from build123d import *

# Parameters (mm, degrees)
PAD009_DEPTH    = 3
POCKET012_DEPTH = 5
SKETCH044_R     = 1.45
POCKET016_DEPTH = 22
FILLET007_R     = 1.5
FILLET015_R     = 0.5


with BuildPart() as part:
    # Sketch032 → Pad009 (new body)
    with BuildSketch(Plane.XY):
        with BuildLine():
            add(Edge.make_bspline(
                [(48.133333, -17.5342), (72.566704, -17.735607), (107.262527, -17.223288), (153.231854, -38.154949)],
                knots=[0, 0, 0, 0, 1, 1, 1, 1], degree=3))
            Line((153.231854, -38.154949), (175.310198, 11.234895))
            add(Edge.make_bspline(
                [(150.875, 88.9625), (150.875, 42.8625), (150.875, 22.157965), (175.310198, 11.234895)],
                knots=[0, 0, 0, 0, 1, 1, 1, 1], degree=3))
            add(Edge.make_bspline(
                [(85.725, 98.4875), (104.775, 98.4875), (104.775, 88.9625), (150.875, 88.9625)],
                knots=[0, 0, 0, 0, 1, 1, 1, 1], degree=3))
            Line((85.725, 98.4875), (66.675, 98.4875))
            add(Edge.make_bspline(
                [(66.675, 98.4875), (58.346897, 98.489647), (52.856461, 97.147667), (48.133333, 95.467873)],
                knots=[0, 0, 0, 0, 1, 1, 1, 1], degree=3))
            Line((48.133333, 95.467873), (48.133333, -17.5342))
        make_face()
    extrude(amount=PAD009_DEPTH)

    # Sketch033 → Pocket012 (cut)
    with BuildSketch(Plane(origin=(0, 0, 0), x_dir=(1, 0, 0), z_dir=(0, 0, -1))):
        Polygon((85.725, -86.475), (105.525, -86.475), (105.525, -81.7125), (143.625, -81.7125), (143.625, -17.457464), (165.732668, -7.574851), (149.57181, 28.577419), (131.568158, 20.529392), (102.96164, 14.448889), (103.848827, 10.275), (85.725, 10.275), align=None)
    extrude(amount=-POCKET012_DEPTH, mode=Mode.SUBTRACT)

    # Sketch044 → Pocket016 (cut)
    with BuildSketch(Plane.XY):
        with Locations((-4.375, -4.375)):
            Circle(SKETCH044_R)
        with Locations((-4.375, 80.575)):
            Circle(SKETCH044_R)
        with Locations((151.401832, -33.366184)):
            Circle(SKETCH044_R)
        with Locations((170.521433, 9.404873)):
            Circle(SKETCH044_R)
        with Locations((147.25, 85.3375)):
            Circle(SKETCH044_R)
        with Locations((43.25, -13.9)):
            Circle(SKETCH044_R)
        with Locations((57.15, 92.085)):
            Circle(SKETCH044_R)
        with Locations((95.25, 92.085)):
            Circle(SKETCH044_R)
        with Locations((95.25, -13.9)):
            Circle(SKETCH044_R)
    extrude(amount=POCKET016_DEPTH, mode=Mode.SUBTRACT)

    # Fillet007
    fillet007_edges = [part.edges().sort_by_distance(p)[0] for p in [
        (153.231854, -38.154949, 1.5),
        (175.310198, 11.234895, 1.5),
        (150.875, 88.9625, 1.5),
    ]]
    fillet(fillet007_edges, radius=FILLET007_R)

    # Fillet015
    fillet015_edges = [part.edges().sort_by_distance(p)[0] for p in [
        (48.133333, -17.5342, 1.5),
        (48.133333, 95.467873, 1.5),
    ]]
    fillet(fillet015_edges, radius=FILLET015_R)


with BuildPart() as part_1:
    # Body008 placement: moved
    add(part.part.moved(Location((0, 0, -15))))


solid = part_1.part
Work out the finished part from the listing and answer in its coordinate system (mm). A direction names the side the tool comes from. Give positions to 0.01 mm unless a question says otherwise; leave off trailing zeros. Loops run counter-clockwise (first coordinate to the right, second up) from the corner with the lowest first, then second, coordinate; pieces in that order, holes last. Notation, with made-up numbers: (0.25, 66.25) -> (8.25, 66.25) arc R11 ccw to (8.25, 70.25) -> close; hole circle Ø10 at (66, -7). An arc over 180 degrees is marked (long way). Use a Markdown table: item, result. Add a question column.
1) Consider line 1 along X through (y, z) = (80.5, -13.55) (3 decimals); line 2 along Y through (x, z) = (147.25, -13.3); line 3 along Y through (x, z) = (140, -14.5). Determine where each line is inside the solid, lowest interval first.
2) For a pull along Y with two mould halves and no side action, classify faces 1 (the flat face through (164.13, -13.775, -13.521)), 2 (the flat face through (82, 31, -15)), 3 (the flat face through (85.725, 37, -14)) as +Y half, -Y half, draft (parallel to the pull), parting line (faces both ways), or undercut.
3) The part is cut by section B-B, the plane z = -14.3. Count the separate pieces of the cut face and the enclosed holes in it, plus the area to 3 significant figures.
4) Which of the six approach directions +Z, -Z, +X, -X, +Y, -Y give full straight-line access (tool end or side, diameter ignored) to faces 4 (the flat face through (143.625, 50, -14)), 5 (the flat face through (48.133, 40, -14))?
5) Each of these flat-tipped pins is pushed along its axis until it touches: P1, Ø0.9, axis at x = 100.5, z = -14, coming from the -Y side; P2, Ø0.9, axis at x = 133.5, z = -13.5, coming from the -Y side; P3, Ø1.7, axis at x = 147.25, y = 85.34, coming from the +Z side. Where does it stop, or does it pass through?
6) The part is cut by section A-A, the plane y = -4. Determine the outline of the cut face in (x, z) (3 decimals), plus the area to 3 significant figures.
Reported:
| question | item | result |
|---|---|---|
| 1 | line 1 | x = 48.133 to 85.725, 143.625 to 150.881 |
| 1 | line 2 | y = -35.52 to -27.54, 15.84 to 83.89, 86.79 to 88.98 |
| 1 | line 3 | y = -32.58 to -24.3, 81.71 to 89.16 |
| 2 | face 1 | -Y half |
| 2 | face 2 | draft |
| 2 | face 3 | undercut |
| 3 | separate pieces | 1 |
| 3 | enclosed holes | 7 |
| 3 | area | 6,630 mm^2 |
| 4 | face 4 | +Z, -Z |
| 4 | face 5 | +Z, -Z, -X, +Y, -Y |
| 5 | P1 | stops at y = -21.44 |
| 5 | P2 | stops at y = -30.34 |
| 5 | P3 | passes through |
| 6 | outline | (48.133, -15) -> (85.725, -15) -> (85.725, -12) -> (48.133, -12) -> close; (160.558, -15) -> (168.5, -15) -> (168.5, -12) -> (160.558, -12) -> close |
| 6 | area | 137 mm^2 |
